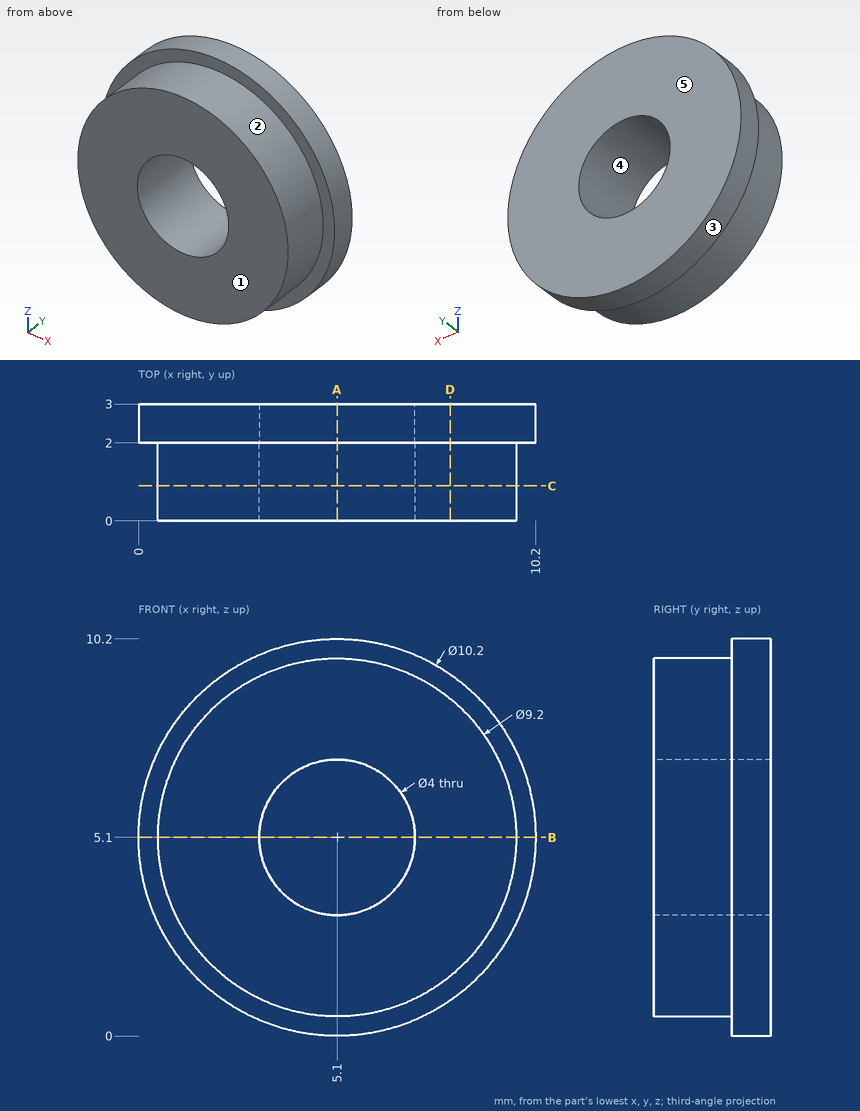
Input: dimensioned drawing with shaded views. Units: mm. Origin: part minimum x, y, z. A direction names the side the tool comes from. Give positions to 0.01 mm unless a question says otherwise; leave off trailing zeros. Write each loop counter-clockwise with the first axis right and the second up, starting at its lowest first coordinate (ties: lowest second). Pieces come first, ordered by that corner, then holes.
1. Section query A-A, the plane x = 5.1. Return loops of the section in (y, z).
2. Line query: probe 1 along Z at (x, y) = (5.1, 0.6); probe 2 along X at (y, z) = (2.2, 5.1). Output: solid intervals per line, ascending.
3. Pin query (flat end, axial travel): P1, Ø6, axis at x = 1, z = 5.5, coming from the -Y side; P2, Ø2.5, axis at x = 5.1, z = 5.1, coming from the +Y side. Return the tip coordinate at first contact, or that it passes through.
4. Reachability of the marked faces 1 and 2 from +Z, -Z, +X, -X, +Y, -Y: full face, straight path, thin tool, end or side. Return the list, or none.
5. Section query C-C, the plane y = 0.9. Return loops of the section in (x, z), then the cut area to 3 significant figures.
6. Section query D-D, the plane x = 8. Return loops of the section in (y, z).
7. Draft query along X for the marked faces 3, 4 and 5. Return one class per face: released by +X, released by -X, zero draft, split by the parting line, or undercut.
8. Section query B-B, the plane z = 5.1. Return loops of the section in (x, y).
Computed:
1. outline: (0, 0.5) - (2, 0.5) - (2, 0) - (3, 0) - (3, 3.1) - (0, 3.1) - close; (0, 7.1) - (3, 7.1) - (3, 10.2) - (2, 10.2) - (2, 9.7) - (0, 9.7) - close
2. probe 1: z = 0.5 to 3.1, 7.1 to 9.7
2. probe 2: x = 0 to 3.1, 7.1 to 10.2
3. P1: stops at y = 0
3. P2: passes through
4. face 1: +Z, -Z, +X, -X, -Y
4. face 2: -Y
5. outline: circle Ø9.2 at (5.1, 5.1); hole circle Ø4 at (5.1, 5.1)
5. area: 53.9 mm2
6. outline: (0, 1.53) - (2, 1.53) - (2, 0.9) - (3, 0.9) - (3, 9.3) - (2, 9.3) - (2, 8.67) - (0, 8.67) - close
7. face 3: split by the parting line
7. face 4: undercut
7. face 5: zero draft
8. outline: (0, 2) - (0.5, 2) - (0.5, 0) - (3.1, 0) - (3.1, 3) - (0, 3) - close; (7.1, 0) - (9.7, 0) - (9.7, 2) - (10.2, 2) - (10.2, 3) - (7.1, 3) - close
